Geometry: see drawing. Coordinates: mm, zero at the bounding-box minimum. Round coordinates to 2 decimals unless told otherwise and drop trailing zeros. Write each loop counter-clockwise with the first axis right and the second up, starting at its lowest first coordinate (ties: lowest second). Pieces come first, ordered by that corner, then holes. Notation, with made-up numbers: M 75.25,-7 L 100.25,-7 A28 cw 100.25,26 Z; hole C -27,72 d4. An arc over 180 degrees is marked long. Use one line per item in the form item = value. Start each with the question number.
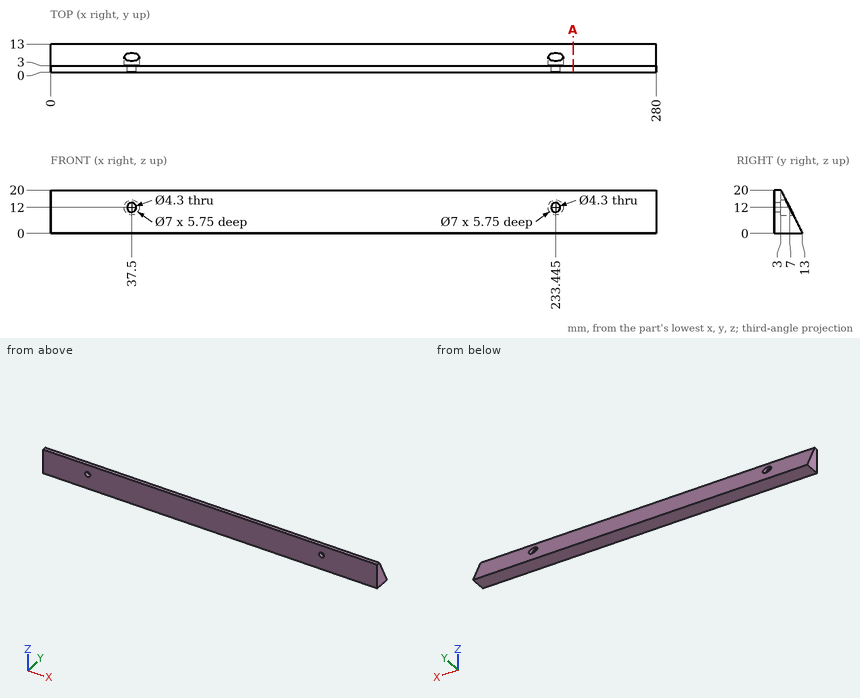
Item 1: Cut plane A-A (x = 241.5). Output: boundary loops of the cut face in (y, z).
Item 2: Ray query, line 1 (X direction, y = 5.75, z = 9.25) (1 decimal); line 2 (X direction, y = 5.3, z = 12) (3 decimals); line 3 (Z direction, x = 37.5, y = 1.3). Return the intervals inside material, ascending. Write a range as from..to.
Item 3: First-contact query: pin 1 (1.5 mm diameter, centred on x = 85, z = 13, fed in from -Y); pin 2 (8 mm diameter, centred on x = 37.5, z = 12, fed in from +Y); pin 3 (5.5 mm diameter, centred on x = 37.5, z = 11, fed in from +Y) (3 decimals); pin 4 (9 mm diameter, centred on x = 233.45, z = 12, fed in from +Y). Flat tips, straight axial feed; report the tip coordinate or a pass-through.
Final values:
q1.outline = M 0,0 L 13,0 L 3,20 L 0,20 Z
q2.line_1 = 0..35.3, 39.7..231.3, 235.6..280
q2.line_2 = 0..34, 41..229.945, 236.945..280
q2.line_3 = 0..9.85, 14.15..20
q3.pin_1 = 0
q3.pin_2 = 9
q3.pin_3 = 8.875
q3.pin_4 = 9.25
